CAD build for the part. Positions are in the model's coordinates, mm. Face numbers are marked on the shaded views. A direction names the side the tool comes from. Round coordinates to 2 decimals unless told otherwise and drop trailing zeros. Order: outer loops, then holes, each group sorted by start corner. A loop starts at its lowest first (then second) coordinate and runs counter-clockwise, first axis right, second up. Notation, with made-up numbers: (-33, 32) - (7, 32) arc R23 cw to (7, 42) - close; hole circle Ø10 at (-12.75, 0). An arc over 180 degrees is marked (long way). Write item = value, one per line.
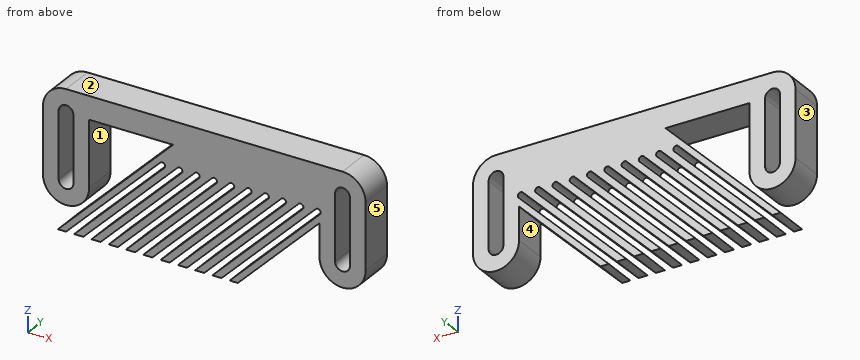
from build123d import *

# Parameters (mm, degrees)
SKETCH1_W           = 177.8
SKETCH1_H           = 76.2
BOSS_EXTRUDE1_DEPTH = 19.05
CUT_EXTRUDE1_DEPTH  = 99.578509321
LPATTERN1_COUNT     = 10
LPATTERN1_PITCH     = 9.525
CUT_EXTRUDE3_DEPTH  = 99.578509321
FILLET1_R           = 12.7
CUT_EXTRUDE4_REACH  = 100.579


with BuildPart() as part:
    # Sketch1 → Boss-Extrude1 (new body)
    with BuildSketch(Plane(origin=(0, 0, 0), x_dir=(1, 0, 0), z_dir=(0, 1, 0))):
        Rectangle(SKETCH1_W, SKETCH1_H)
    extrude(amount=BOSS_EXTRUDE1_DEPTH)

    # Sketch2 → Cut-Extrude1 (cut, through all)
    with BuildSketch(Plane(origin=(0, 19.05, 0), x_dir=(1, 0, 0), z_dir=(0, 1, 0))):
        with BuildLine():
            Line((-76.2, 38.1), (-24.277467985, -13.822532015))
            ThreePointArc((-24.277467985, -13.822532015), (-22.032403955, -13.822532015), (-22.032403955, -11.577467985))
            Line((-22.032403955, -11.577467985), (-71.709871939, 38.1))
            Line((-71.709871939, 38.1), (-76.2, 38.1))
        make_face()
    cut_extrude1 = extrude(amount=-CUT_EXTRUDE1_DEPTH, mode=Mode.SUBTRACT)

    # LPattern1: Cut-Extrude1 ×10
    with Locations(*[(i * LPATTERN1_PITCH, 0, 0) for i in range(1, LPATTERN1_COUNT)]):
        add(cut_extrude1, mode=Mode.SUBTRACT)

    # Sketch3 → Cut-Extrude3 (cut, through all)
    with BuildSketch(Plane(origin=(0, 19.05, 0), x_dir=(1, 0, 0), z_dir=(0, 1, 0))):
        with BuildLine():
            Line((-72.136, 11.176), (-72.136, -25.4))
            ThreePointArc((-72.136, -25.4), (-76.2, -29.464), (-80.264, -25.4))
            Line((-80.264, -25.4), (-80.264, 11.176))
            ThreePointArc((-80.264, 11.176), (-76.2, 15.24), (-72.136, 11.176))
        make_face()
        with BuildLine():
            Line((80.264, 11.176), (80.264, -25.4))
            ThreePointArc((80.264, -25.4), (76.2, -29.464), (72.136, -25.4))
            Line((72.136, -25.4), (72.136, 11.176))
            ThreePointArc((72.136, 11.176), (76.2, 15.24), (80.264, 11.176))
        make_face()
    extrude(amount=-CUT_EXTRUDE3_DEPTH, mode=Mode.SUBTRACT)

    # Fillet1
    fillet1_edges = [part.edges().sort_by_distance(p)[0] for p in [
        (88.9, 9.525, 38.1),
        (-88.9, 9.525, 38.1),
    ]]
    fillet(fillet1_edges, radius=FILLET1_R)

    # Sketch5 → Cut-Extrude4 (cut, up to next)
    with BuildSketch(Plane(origin=(0, 19.05, 0), x_dir=(1, 0, 0), z_dir=(0, 1, 0)), mode=Mode.PRIVATE) as cut_extrude4_sk1:
        with BuildLine():
            Line((-88.9, 38.1), (-88.9, 11.176))
            ThreePointArc((-88.9, 11.176), (-76.2, 23.876), (-63.5, 11.176))
            Line((-63.5, 11.176), (-63.5, -25.4))
            Line((-63.5, -25.4), (-17.190128061, -25.4))
            Line((-17.190128061, -25.4), (-80.690128061, 38.1))
            Line((-80.690128061, 38.1), (-88.9, 38.1))
        make_face()
    cut_extrude4_tool1 = extrude(cut_extrude4_sk1.sketch, amount=-CUT_EXTRUDE4_REACH, mode=Mode.PRIVATE) & part.part
    # Sketch5 → Cut-Extrude4 (cut, up to next)
    with BuildSketch(Plane(origin=(0, 19.05, 0), x_dir=(1, 0, 0), z_dir=(0, 1, 0)), mode=Mode.PRIVATE) as cut_extrude4_sk2:
        with BuildLine():
            Line((88.9, 38.1), (88.9, 11.176))
            ThreePointArc((88.9, 11.176), (76.2, 23.876), (63.5, 11.176))
            Line((63.5, 11.176), (63.5, -6.894743879))
            Line((63.5, -6.894743879), (18.505256121, 38.1))
            Line((18.505256121, 38.1), (88.9, 38.1))
        make_face()
    cut_extrude4_tool2 = extrude(cut_extrude4_sk2.sketch, amount=-CUT_EXTRUDE4_REACH, mode=Mode.PRIVATE) & part.part
    add(cut_extrude4_tool1.solids().sort_by_distance((-54.694692, 19.05, 2.076877))[0], mode=Mode.SUBTRACT)
    add(cut_extrude4_tool2.solids().sort_by_distance((56.766727, 19.05, -24.977603))[0], mode=Mode.SUBTRACT)


solid = part.part
(1) Band-saw the part on A-A on x = 40. List the corners of the cut face in (y, z) (3 decimals).
Solved:
outline = (0, -16.605) - (19.05, -16.605) - (19.05, -12.115) - (0, -12.115) - close; (0, -7.625) - (19.05, -7.625) - (19.05, -2.59) - (0, -2.59) - close; (0, 1.9) - (19.05, 1.9) - (19.05, 6.935) - (0, 6.935) - close; (0, 11.425) - (19.05, 11.425) - (19.05, 38.1) - (0, 38.1) - close
(2) Band-saw the part on C-C on x = -68.5. List the corners of the cut face in (y, z), plus the area to 3 significant figures.
Solved:
outline = (0, -38.1) - (19.05, -38.1) - (19.05, -34.89) - (0, -34.89) - close; (0, -30.4) - (19.05, -30.4) - (19.05, -25.91) - (0, -25.91) - close; (0, -21.28) - (19.05, -21.28) - (19.05, 38.1) - (0, 38.1) - close
area = 1,280 mm²
(3) Pull direction X, two halves, no side cores. Call the marked faces 3, 4 and 5: released by +X, released by -X, zero draft, split by the parting line, or undercut.
Solved:
face_3 = released by -X
face_4 = undercut
face_5 = released by +X
(4) Probe line 1 along Z through (x, y) = (-7, 1) (3 decimals); line 2 along Z through (x, y) = (-57.5, 14.25) (3 decimals); line 3 along Z through (x, y) = (-74, 2.25). List the from-to ranges inside material, lowest first.
Solved:
line_1 = -35.575 to -30.54, -26.05 to -21.015, -16.525 to -11.49, -7 to -1.965, 2.525 to 7.56, 12.05 to 38.1
line_2 = -38.1 to -33.415, -28.925 to -23.89, -19.4 to -14.91, 25.4 to 38.1
line_3 = -35.9 to -31.41, -23.68 to -14.59, 28.82 to 38.1
(5) Drop flat-ended pins along their axis: pin 1 (1 mm diameter, centred on y = 12.5, z = -17, fed in from +X); pin 2 (1 mm diameter, centred on y = 17, z = -15.5, fed in from -X). Give the stop position or say it passes through.
Solved:
pin_1 = 87.73
pin_2 = -88.31
(6) Band-saw the part on B-B on z = 20. List the corners of the cut face in (x, y).
Solved:
outline = (-88.9, 0) - (-80.26, 0) - (-80.26, 19.05) - (-88.9, 19.05) - close; (-72.14, 0) - (-63.5, 0) - (-63.5, 19.05) - (-72.14, 19.05) - close; (-22.59, 0) - (72.14, 0) - (72.14, 19.05) - (-22.59, 19.05) - close; (80.26, 0) - (88.9, 0) - (88.9, 19.05) - (80.26, 19.05) - close
(7) Tool access for the marked faces 1 and 2: list every direction of +Z, -Z, +X, -X, +Y, -Y with a clear straight run to the whole face (end or side of a thin tool).
Solved:
face_1 = +Y, -Y
face_2 = +Z, +X, -X, +Y, -Y
(8) Band-saw the part on D-D on y = 14. Count the separate pieces of the cut face and the enclosed holes in it, plus the area to 3 significant figures.
Solved:
separate_pieces = 1
enclosed_holes = 2
area = 7,660 mm²
